Here's how the part is built. I have some questions about the finished solid (model axes, mm). A direction names the side the tool comes from. Coordinates: 2 decimals unless noted, no trailing zeros. Loops run counter-clockwise (first coordinate to the right, second up) from the corner with the lowest first, then second, coordinate; pieces in that order, holes last. Notation, with made-up numbers: (-38.5, 56) -> (-14.5, 56) arc R20 ccw to (-14.5, 85) -> close; hole circle Ø5 at (-13.5, 37.5). An arc over 180 degrees is marked (long way). Answer as a JSON object with one key per item and string values. Group by question number.
Q1. I want a section at B-B on x = 57.15. Write out the boundary of the cut face in (y, z) (3 decimals), then the cut area to 3 significant figures.
Q2. I want a section at D-D on x = 23. Write out the boundary of the cut face in (y, z) (3 decimals).
Q3. Thinking about a two-plate mould opening in X: for faces 3 (the flat face through (42, -65, 7.62)), 4 (the cylindrical face through (-72.8, -22.93, 6.01)), 5 (the cylindrical face through (-75.71, -23.84, 3.76)), which applies, released by +X, released by -X, zero draft, split by the parting line, or undercut?
Q4. I'm going to push flat-ended pins straight in: pin 1 (22 mm diameter, centred on x = 57.15, y = 0, fed in from +Z) (3 decimals); pin 2 (1.5 mm diameter, centred on y = 42, z = 5.5, fed in from -X); pin 3 (2.5 mm diameter, centred on x = 0, y = -9.525, fed in from -Z); pin 4 (1.5 mm diameter, centred on x = -63.5, z = 2, fed in from +Y). Where does each tip first touch, or does it pass through?
Q5. I need wall thicknesses on line 1 (Y direction, x = 0, z = 1.7) (1 decimal); line 2 (X direction, y = -1, z = 6.25); line 3 (Y direction, x = 0, z = 5.75) (1 decimal). Which ranges of each line are inside material? Lowest first, please.
Q6. I want a section at A-A on z = 6. Count the separate pieces of the cut face and the enclosed holes in it, then the cut area to 3 significant figures.
Q7. On a 3-axis mill with a long thin cutter (end or side, diameter ignored), from which of +Z, -Z, +X, -X, +Y, -Y can I reach the whole of each face in a straight line? I mean faces 1 (the cylindrical face through (-2.06, 47.85, 2.25)), 2 (the flat face through (-33, 33, 4.445)). Say none if no direction works.
```python
from build123d import *

# Parameters (mm, degrees)
SKETCH1_R             = 44.323
BOSS_EXTRUDE1_DEPTH   = 7.62
SKETCH1_R_2           = 79.375
SKETCH1_R_3           = 76.327
BOSS_EXTRUDE1_2_DEPTH = 7.62
SKETCH1_3_R           = 76.327
SKETCH1_3_R_2         = 44.323
BOSS_EXTRUDE2_DEPTH   = 4.445
CUT_EXTRUDE1_REACH    = 114.512
SKETCH2_R             = 1.5875
CUT_EXTRUDE2_REACH    = 114.341
SKETCH3_R             = 9.525


with BuildPart() as part:
    # Sketch1 → Boss-Extrude1 (new body)
    with BuildSketch(Plane.XY):
        with Locations(Location((0, 0, 0), (0, 0, 180))):
            Circle(SKETCH1_R)
    extrude(amount=BOSS_EXTRUDE1_DEPTH)



with BuildPart() as body_2:
    # Sketch1 → Boss-Extrude1 2 (new body)
    with BuildSketch(Plane.XY):
        with Locations(Location((0, 0, 0), (0, 0, 180))):
            Circle(SKETCH1_R_2)
        with Locations(Location((0, 0, 0), (0, 0, 180))):
            Circle(SKETCH1_R_3, mode=Mode.SUBTRACT)
    extrude(amount=BOSS_EXTRUDE1_2_DEPTH)


with BuildPart() as part_1:
    add(part.part)

    add(body_2.part)  # Boss-Extrude2 merges body 2
    # Sketch1_3 → Boss-Extrude2 (add)
    with BuildSketch(Plane.XY):
        with Locations(Location((0, 0, 0), (0, 0, 180))):
            Circle(SKETCH1_3_R)
        with Locations(Location((0, 0, 0), (0, 0, 180))):
            Circle(SKETCH1_3_R_2, mode=Mode.SUBTRACT)
    extrude(amount=BOSS_EXTRUDE2_DEPTH)

    # Sketch2 → Cut-Extrude1 (cut, up to next)
    with BuildSketch(Plane.XY.offset(7.62), mode=Mode.PRIVATE) as cut_extrude1_sk1:
        with Locations((0, 9.525)):
            Circle(SKETCH2_R)
    cut_extrude1_tool1 = extrude(cut_extrude1_sk1.sketch, amount=-CUT_EXTRUDE1_REACH, mode=Mode.PRIVATE) & part_1.part
    # Sketch2 → Cut-Extrude1 (cut, up to next)
    with BuildSketch(Plane.XY.offset(7.62), mode=Mode.PRIVATE) as cut_extrude1_sk2:
        with Locations((8.248891971, 4.7625)):
            Circle(SKETCH2_R)
    cut_extrude1_tool2 = extrude(cut_extrude1_sk2.sketch, amount=-CUT_EXTRUDE1_REACH, mode=Mode.PRIVATE) & part_1.part
    # Sketch2 → Cut-Extrude1 (cut, up to next)
    with BuildSketch(Plane.XY.offset(7.62), mode=Mode.PRIVATE) as cut_extrude1_sk3:
        with Locations((8.248891971, -4.7625)):
            Circle(SKETCH2_R)
    cut_extrude1_tool3 = extrude(cut_extrude1_sk3.sketch, amount=-CUT_EXTRUDE1_REACH, mode=Mode.PRIVATE) & part_1.part
    # Sketch2 → Cut-Extrude1 (cut, up to next)
    with BuildSketch(Plane.XY.offset(7.62), mode=Mode.PRIVATE) as cut_extrude1_sk4:
        with Locations((0, -9.525)):
            Circle(SKETCH2_R)
    cut_extrude1_tool4 = extrude(cut_extrude1_sk4.sketch, amount=-CUT_EXTRUDE1_REACH, mode=Mode.PRIVATE) & part_1.part
    # Sketch2 → Cut-Extrude1 (cut, up to next)
    with BuildSketch(Plane.XY.offset(7.62), mode=Mode.PRIVATE) as cut_extrude1_sk5:
        with Locations((-8.248891971, -4.7625)):
            Circle(SKETCH2_R)
    cut_extrude1_tool5 = extrude(cut_extrude1_sk5.sketch, amount=-CUT_EXTRUDE1_REACH, mode=Mode.PRIVATE) & part_1.part
    # Sketch2 → Cut-Extrude1 (cut, up to next)
    with BuildSketch(Plane.XY.offset(7.62), mode=Mode.PRIVATE) as cut_extrude1_sk6:
        with Locations((-8.248891971, 4.7625)):
            Circle(SKETCH2_R)
    cut_extrude1_tool6 = extrude(cut_extrude1_sk6.sketch, amount=-CUT_EXTRUDE1_REACH, mode=Mode.PRIVATE) & part_1.part
    add(cut_extrude1_tool1.solids().sort_by_distance((0, 9.525, 7.62))[0], mode=Mode.SUBTRACT)
    add(cut_extrude1_tool2.solids().sort_by_distance((8.248892, 4.7625, 7.62))[0], mode=Mode.SUBTRACT)
    add(cut_extrude1_tool3.solids().sort_by_distance((8.248892, -4.7625, 7.62))[0], mode=Mode.SUBTRACT)
    add(cut_extrude1_tool4.solids().sort_by_distance((0, -9.525, 7.62))[0], mode=Mode.SUBTRACT)
    add(cut_extrude1_tool5.solids().sort_by_distance((-8.248892, -4.7625, 7.62))[0], mode=Mode.SUBTRACT)
    add(cut_extrude1_tool6.solids().sort_by_distance((-8.248892, 4.7625, 7.62))[0], mode=Mode.SUBTRACT)

    # Sketch3 → Cut-Extrude2 (cut, up to next)
    with BuildSketch(Plane.XY.offset(4.445), mode=Mode.PRIVATE) as cut_extrude2_sk1:
        with Locations((0, 57.15)):
            Circle(SKETCH3_R)
    cut_extrude2_tool1 = extrude(cut_extrude2_sk1.sketch, amount=-CUT_EXTRUDE2_REACH, mode=Mode.PRIVATE) & part_1.part
    # Sketch3 → Cut-Extrude2 (cut, up to next)
    with BuildSketch(Plane.XY.offset(4.445), mode=Mode.PRIVATE) as cut_extrude2_sk2:
        with Locations((57.15, 0)):
            Circle(SKETCH3_R)
    cut_extrude2_tool2 = extrude(cut_extrude2_sk2.sketch, amount=-CUT_EXTRUDE2_REACH, mode=Mode.PRIVATE) & part_1.part
    # Sketch3 → Cut-Extrude2 (cut, up to next)
    with BuildSketch(Plane.XY.offset(4.445), mode=Mode.PRIVATE) as cut_extrude2_sk3:
        with Locations((0, -57.15)):
            Circle(SKETCH3_R)
    cut_extrude2_tool3 = extrude(cut_extrude2_sk3.sketch, amount=-CUT_EXTRUDE2_REACH, mode=Mode.PRIVATE) & part_1.part
    # Sketch3 → Cut-Extrude2 (cut, up to next)
    with BuildSketch(Plane.XY.offset(4.445), mode=Mode.PRIVATE) as cut_extrude2_sk4:
        with Locations((-57.15, 0)):
            Circle(SKETCH3_R)
    cut_extrude2_tool4 = extrude(cut_extrude2_sk4.sketch, amount=-CUT_EXTRUDE2_REACH, mode=Mode.PRIVATE) & part_1.part
    add(cut_extrude2_tool1.solids().sort_by_distance((0, 57.15, 4.445))[0], mode=Mode.SUBTRACT)
    add(cut_extrude2_tool2.solids().sort_by_distance((57.15, 0, 4.445))[0], mode=Mode.SUBTRACT)
    add(cut_extrude2_tool3.solids().sort_by_distance((0, -57.15, 4.445))[0], mode=Mode.SUBTRACT)
    add(cut_extrude2_tool4.solids().sort_by_distance((-57.15, 0, 4.445))[0], mode=Mode.SUBTRACT)


solid = part_1.part
```
Result set:
{
 "1": {"outline": "(-55.084, 0) -> (-9.525, 0) -> (-9.525, 4.445) -> (-50.593, 4.445) -> (-50.593, 7.62) -> (-55.084, 7.62) -> close; (9.525, 0) -> (55.084, 0) -> (55.084, 7.62) -> (50.593, 7.62) -> (50.593, 4.445) -> (9.525, 4.445) -> close", "area": "434 mm²"},
 "2": {"outline": "(-75.97, 0) -> (75.97, 0) -> (75.97, 7.62) -> (72.779, 7.62) -> (72.779, 4.445) -> (37.888, 4.445) -> (37.888, 7.62) -> (-37.888, 7.62) -> (-37.888, 4.445) -> (-72.779, 4.445) -> (-72.779, 7.62) -> (-75.97, 7.62) -> close"},
 "3": {"face 3": "zero draft", "face 4": "undercut", "face 5": "split by the parting line"},
 "4": {"pin 1": "stops at z = 4.445", "pin 2": "stops at x = -67.81", "pin 3": "passes through", "pin 4": "stops at y = 48.61"},
 "5": {"line 1": "y = -79.4 to -66.7, -47.6 to -11.1, -7.9 to 7.9, 11.1 to 47.6, 66.7 to 79.4", "line 2": "x = -79.37 to -76.32, -44.31 to 44.31, 76.32 to 79.37", "line 3": "y = -79.4 to -76.3, -44.3 to -11.1, -7.9 to 7.9, 11.1 to 44.3, 76.3 to 79.4"},
 "6": {"separate pieces": "2", "enclosed holes": "7", "area": "7,620 mm²"},
 "7": {"face 1": "+Z, -Z", "face 2": "+Z"}
}
